```python
from build123d import *

# Parameters (mm, degrees)
F1_DEPTH = 20
F2_W     = 8
F2_H     = 8
F2_R     = 3
F3_DEPTH = 10
F4_R     = 2.25
F5_DEPTH = 18.5


with BuildPart() as f1:
    # F0 (on Top) → F1 (new body)
    with BuildSketch(Plane.XY):
        Polygon((0, -3.464102), (3, -1.732051), (3, 1.732051), (0, 3.464102), (-3, 1.732051), (-3, -1.732051), align=None)
    extrude(amount=F1_DEPTH)

    # F2 (on face) → F3 (cut)
    with BuildSketch(Plane.XY.offset(20)):
        Rectangle(F2_W, F2_H)
        Circle(F2_R, mode=Mode.SUBTRACT)
    extrude(amount=-F3_DEPTH, mode=Mode.SUBTRACT)

    # F4 (on face) → F5 (cut)
    with BuildSketch(Plane.XY.offset(20)):
        Circle(F4_R)
    extrude(amount=-F5_DEPTH, mode=Mode.SUBTRACT)


solid = f1.part
```
Could you check a few things on this model? Use its own coordinates, in mm. A direction names the side the tool comes from. Give positions to 0.01 mm unless a question says otherwise; leave off trailing zeros. Write each loop counter-clockwise with the first axis right and the second up, starting at its lowest first coordinate (ties: lowest second). Pieces come first, ordered by that corner, then holes. Notation, with made-up numbers: (70.5, -31) - (112.5, -31) arc R27 cw to (112.5, 8) - close; hole circle Ø7 at (85, 2.25). An arc over 180 degrees is marked (long way). One line per item, written item: value. Start each with the question number.
Item 1: I'm going to push a flat-ended pin straight in: pin 1 (3.5 mm diameter, centred on x = 0, y = 0, fed in from +Z). Where does the tip first touch, or does it pass through?
Item 2: Imagine slicing it at A-A, the plane z = 6.75. List the corners of the cut face in (x, y) for me.
Item 3: Which directions (+Z, -Z, +X, -X, +Y, -Y) give clear straight access to the entire face, cutting with the end or side of a thin tool? Please do faces 1 (the face through (0, 0, 1.5)), 2 (the face through (-0.24, 3.15, 10)), 3 (the face through (1.5, -2.6, 4.9)).
Item 4: If we mould it in two halves opening along X, with no side actions, what happens to faces 4 (the face through (0, 0, 0)), 5 (the face through (3, 0, 5)), 6 (the face through (-0.29, 2.23, 10.88)), 7 (the face through (-1.5, -2.6, 4.9))? For each: +X half, -X half, draft (parallel to the pull), parting line (faces both ways), or undercut.
Item 5: Imagine slicing it at C-C, the plane x = 1. List the corners of the cut face in (y, z) for me.
Item 6: Imagine slicing it at B-B, the plane y = 1.5. List the corners of the cut face in (x, z) for me, and give its area (3 significant figures).
Item 7: Imagine slicing it at D-D, the plane z = 18. List the corners of the cut face in (x, y) for me.
Item 8: Please list where these lines run through material, in increasing order: line 1 (Y direction, x = 0, z = 15.75); line 2 (Z direction, x = 2.75, y = -1.75); line 3 (Y direction, x = 2, z = 16.75). Write a range as from..to.
Geometry says:
1. pin 1: z = 1.5
2. outline: (-3, -1.73) - (0, -3.46) - (3, -1.73) - (3, 1.73) - (0, 3.46) - (-3, 1.73) - close; hole circle Ø4.5 at (0, 0)
3. face 1: +Z
3. face 2: +Z, +Y
3. face 3: +Z, -Z, +X, -Y
4. face 4: draft
4. face 5: +X half
4. face 6: undercut
4. face 7: -X half
5. outline: (-2.89, 0) - (2.89, 0) - (2.89, 10) - (2.83, 10) - (2.83, 20) - (2.02, 20) - (2.02, 1.5) - (-2.02, 1.5) - (-2.02, 20) - (-2.83, 20) - (-2.83, 10) - (-2.89, 10) - close
6. outline: (-3, 0) - (3, 0) - (3, 10) - (2.6, 10) - (2.6, 20) - (1.68, 20) - (1.68, 1.5) - (-1.68, 1.5) - (-1.68, 20) - (-2.6, 20) - (-2.6, 10) - (-3, 10) - close
6. area: 49.9 mm^2
7. outline: circle Ø6 at (0, 0); hole circle Ø4.5 at (0, 0)
8. line 1: -3..-2.25, 2.25..3
8. line 2: 0..10
8. line 3: -2.24..-1.03, 1.03..2.24
